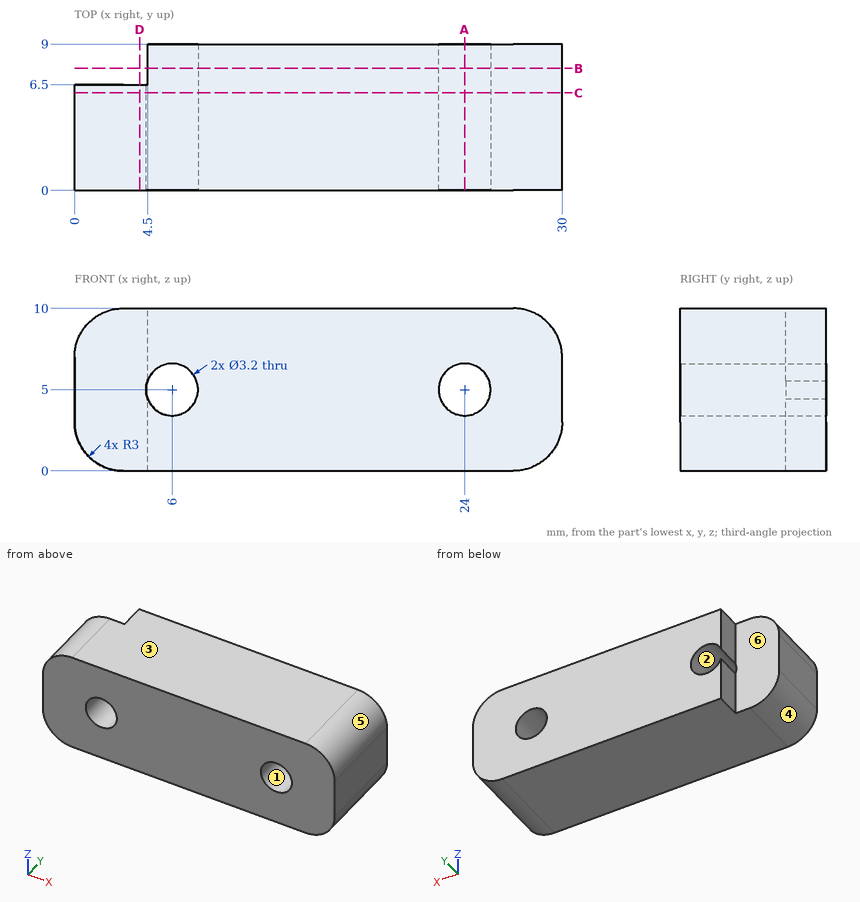
Study the drawing (mm; zero at the part's minimum x, y, z) and answer. A direction names the side the tool comes from. Give positions to 0.01 mm unless a question says otherwise; leave off trailing zeros. Loops run counter-clockwise (first coordinate to the right, second up) from the corner with the lowest first, then second, coordinate; pieces in that order, holes last. Notation, with made-up numbers: (19, -12.5) -> (44, -12.5) arc R27 cw to (44, 15.5) -> close; hole circle Ø2 at (68.25, 4). An arc over 180 degrees is marked (long way). Write item = value, one per line. Start each with the question number.
(1) Find the intervals of material crossed by probe 1 along Z at (x, y) = (6, 6.5); probe 2 along Z at (x, y) = (25.25, 6.5); probe 3 along Y at (x, z) = (3.5, 5.75), in increasing order. Write a range as from..to.
(2) Find section B-B on y = 7.5. Give the vertices of the cut face in (x, z), and give its area (3 significant figures).
(3) Find section A-A on x = 24. Give the vertices of the cut face in (y, z), and give its area (3 significant figures).
(4) Which of the six approach directions +Z, -Z, +X, -X, +Y, -Y give full straight-line access (tool end or side, diameter ignored) to the marked faces 5 and 6?
(5) Find section C-C on y = 6. Give the vertices of the cut face in (x, z).
(6) Given pin 1 Ø5 at (x, z) = (24, 5) entering from +Y; pin 2 Ø0.8 at (y, z) = (7.5, 2) entering from -X; pin 3 Ø2 at (x, z) = (1, 3.5) entering from +Y, each flat-ended and moving along its own axis, determine where each tip first touches the part or whether it passes through.
(7) Find section D-D on x = 4. Give the vertices of the cut face in (y, z).
(8) The mould has two halves that part along X. Classify the marked faces 1, 2, 3 and 4: +X half, -X half, draft (parallel to the pull), parting line (faces both ways), or undercut.
From the geometry:
q1.probe_1 = 0..3.4, 6.6..10
q1.probe_2 = 0..4, 6..10
q1.probe_3 = 0..6.5
q2.outline = (4.5, 0) -> (27, 0) arc R3 ccw to (30, 3) -> (30, 7) arc R3 ccw to (27, 10) -> (4.5, 10) -> (4.5, 5.56) arc R1.6 cw (long way) to (4.5, 4.44) -> close; hole circle Ø3.2 at (24, 5)
q2.area = 235 mm^2
q3.outline = (0, 0) -> (9, 0) -> (9, 3.4) -> (0, 3.4) -> close; (0, 6.6) -> (9, 6.6) -> (9, 10) -> (0, 10) -> close
q3.area = 61.2 mm^2
q4.face_5 = +Z, +X, +Y, -Y
q4.face_6 = +Z, -Z, -X, +Y
q5.outline = (0, 3) arc R3 ccw to (3, 0) -> (27, 0) arc R3 ccw to (30, 3) -> (30, 7) arc R3 ccw to (27, 10) -> (3, 10) arc R3 ccw to (0, 7) -> close; hole circle Ø3.2 at (6, 5); hole circle Ø3.2 at (24, 5)
q6.pin_1 = 9
q6.pin_2 = 4.5
q6.pin_3 = 6.5
q7.outline = (0, 0) -> (6.5, 0) -> (6.5, 10) -> (0, 10) -> close
q8.face_1 = undercut
q8.face_2 = undercut
q8.face_3 = draft
q8.face_4 = -X half
